Job drawing, mm, ordinate dimensions from the low corner. One solid piece. Round coordinates to 2 decimals unless told otherwise and drop trailing zeros. Order: outer loops, then holes, each group sorted by start corner. A loop starts at its lowest first (then second) coordinate and runs counter-clockwise, first axis right, second up. Notation, with made-up numbers: (83, 46) -> (90, 46) arc R14 cw to (90, 51) -> close; hole circle Ø2 at (34.25, -15). An arc over 180 degrees is marked (long way). Use CSV: the item, a comma, the result in double quotes.
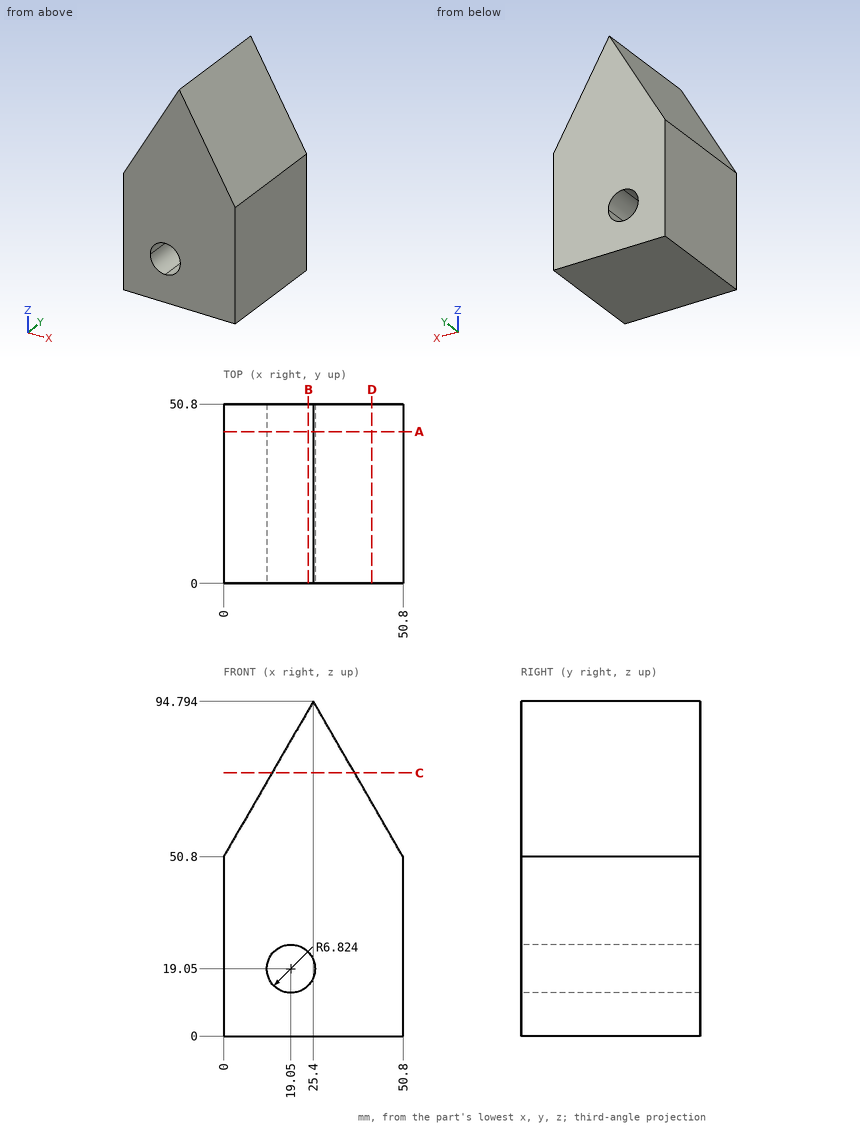
(1) Cut at B-B, the plane x = 24. Give the cut face in (y, z), then the cut area to 4 significant figures.
Reply:
outline,"(0, 0) -> (50.8, 0) -> (50.8, 14.35) -> (0, 14.35) -> close; (0, 23.75) -> (50.8, 23.75) -> (50.8, 92.37) -> (0, 92.37) -> close"
area,"4,215 mm2"
(2) Drop a flat-ended pin along its axis: P1, Ø1, axis at y = 11.5, z = 64, coming from the -X side. Give the stop position or say it passes through.
Reply:
P1,"x = 7.33"
(3) Probe probe 1 along X at (y, z) = (4, 16) (1 decimal); probe 2 along Z at (x, y) = (21.5, 40); probe 3 along X at (y, z) = (45.5, 74.5). List the from-to ranges inside material, lowest first. Write a range as [from, to].
Reply:
probe 1,"[0, 12.9], [25.2, 50.8]"
probe 2,"[0, 12.68], [25.42, 88.04]"
probe 3,"[13.68, 37.12]"
(4) Cut at A-A, the plane y = 43. Give the cut face in (x, z), then the cut area to 3 significant figures.
Reply:
outline,"(0, 0) -> (50.8, 0) -> (50.8, 50.8) -> (25.4, 94.79) -> (0, 50.8) -> close; hole (12.23, 19.05) arc R6.82 ccw to (19.05, 12.23) arc R6.82 ccw to (25.87, 19.05) arc R6.82 ccw to (19.05, 25.87) arc R6.82 ccw to start"
area,"3,550 mm2"
(5) Cut at D-D, the plane x = 42. Give the cut face in (y, z).
Reply:
outline,"(0, 0) -> (50.8, 0) -> (50.8, 66.04) -> (0, 66.04) -> close"
(6) Cut at C-C, the plane z = 74.5. Give the cut face in (x, y).
Reply:
outline,"(13.68, 0) -> (37.12, 0) -> (37.12, 50.8) -> (13.68, 50.8) -> close"
